```python
from build123d import *

# Parameters (mm, degrees)
SKETCH1_W           = 247.82
SKETCH1_H           = 120.12
SKETCH1_R           = 1.6
SKETCH1_H_2         = 10.57
SKETCH1_H_3         = 1.8
BOSS_EXTRUDE1_DEPTH = 4
SKETCH1_5_W         = 247.82
SKETCH1_5_H         = 1.8
BOSS_EXTRUDE2_DEPTH = 0.8
SKETCH1_6_W         = 247.82
SKETCH1_6_H         = 10.57
BOSS_EXTRUDE3_DEPTH = 1.4
SKETCH2_R           = 2.75
CUT_EXTRUDE1_DEPTH  = 2.9
CUT_EXTRUDE2_REACH  = 287.106
FILLET1_R           = 3


with BuildPart() as part:
    # Sketch1 → Boss-Extrude1 (new body)
    # profile 1 of 5: a face of its own
    with BuildSketch(Plane(origin=(0, 0, 0), x_dir=(1, 0, 0), z_dir=(0, 1, 0))):
        with Locations((126.21, -61.86)):
            Rectangle(SKETCH1_W, SKETCH1_H)
        with Locations(Location((8, -111.92, 0), (0, 0, 270))):
            Circle(SKETCH1_R, mode=Mode.SUBTRACT)
        with Locations(Location((244.42, -111.92, 0), (0, 0, 270))):
            Circle(SKETCH1_R, mode=Mode.SUBTRACT)
        with Locations(Location((8, -61.92, 0), (0, 0, 270))):
            Circle(SKETCH1_R, mode=Mode.SUBTRACT)
        with Locations(Location((8, -8, 0), (0, 0, 270))):
            Circle(SKETCH1_R, mode=Mode.SUBTRACT)
        with Locations(Location((63.11, -8, 0), (0, 0, 270))):
            Circle(SKETCH1_R, mode=Mode.SUBTRACT)
        with Locations(Location((244.42, -61.92, 0), (0, 0, 270))):
            Circle(SKETCH1_R, mode=Mode.SUBTRACT)
        with Locations(Location((126.21, -8, 0), (0, 0, 270))):
            Circle(SKETCH1_R, mode=Mode.SUBTRACT)
        with Locations(Location((189.31, -8, 0), (0, 0, 270))):
            Circle(SKETCH1_R, mode=Mode.SUBTRACT)
        with Locations(Location((244.42, -8, 0), (0, 0, 270))):
            Circle(SKETCH1_R, mode=Mode.SUBTRACT)
    # profile 2 of 5: a face of its own
    with BuildSketch(Plane(origin=(0, 0, 0), x_dir=(1, 0, 0), z_dir=(0, 1, 0))):
        Polygon((252.42, 0), (250.12, 0), (250.12, -1.8), (250.12, -121.92), (250.12, -132.49), (252.42, -132.49), align=None)
    # profile 3 of 5: a face of its own
    with BuildSketch(Plane(origin=(0, 0, 0), x_dir=(1, 0, 0), z_dir=(0, 1, 0))):
        with Locations((126.21, -127.205)):
            Rectangle(SKETCH1_W, SKETCH1_H_2)
    # profile 4 of 5: a face of its own
    with BuildSketch(Plane(origin=(0, 0, 0), x_dir=(1, 0, 0), z_dir=(0, 1, 0))):
        Polygon((2.3, 0), (0, 0), (0, -132.49), (2.3, -132.49), (2.3, -121.92), (2.3, -1.8), align=None)
    # profile 5 of 5: a face of its own
    with BuildSketch(Plane(origin=(0, 0, 0), x_dir=(1, 0, 0), z_dir=(0, 1, 0))):
        with Locations((126.21, -0.9)):
            Rectangle(SKETCH1_W, SKETCH1_H_3)
    extrude(amount=BOSS_EXTRUDE1_DEPTH)

    # Sketch1<5> → Boss-Extrude2 (add)
    with BuildSketch(Plane(origin=(0, 0, 0), x_dir=(1, 0, 0), z_dir=(0, 1, 0))):
        Polygon((2.3, 0), (0, 0), (0, -132.49), (2.3, -132.49), (2.3, -121.92), (2.3, -1.8), align=None)
        with Locations((126.21, -0.9)):
            Rectangle(SKETCH1_5_W, SKETCH1_5_H)
        Polygon((252.42, 0), (250.12, 0), (250.12, -1.8), (250.12, -121.92), (250.12, -132.49), (252.42, -132.49), align=None)
    extrude(amount=-BOSS_EXTRUDE2_DEPTH)

    # Sketch1<6> → Boss-Extrude3 (add)
    with BuildSketch(Plane(origin=(0, 0, 0), x_dir=(1, 0, 0), z_dir=(0, 1, 0))):
        with Locations((126.21, -127.205)):
            Rectangle(SKETCH1_6_W, SKETCH1_6_H)
    extrude(amount=BOSS_EXTRUDE3_DEPTH)

    # Sketch2 → Cut-Extrude1 (cut)
    with BuildSketch(Plane(origin=(0, 4, 0), x_dir=(1, 0, 0), z_dir=(0, 1, 0))):
        with Locations(Location((8, -8, 0), (0, 0, 270))):
            Circle(SKETCH2_R)
        with Locations(Location((63.11, -8, 0), (0, 0, 270))):
            Circle(SKETCH2_R)
        with Locations(Location((126.21, -8, 0), (0, 0, 270))):
            Circle(SKETCH2_R)
        with Locations(Location((189.31, -8, 0), (0, 0, 270))):
            Circle(SKETCH2_R)
        with Locations(Location((244.42, -8, 0), (0, 0, 270))):
            Circle(SKETCH2_R)
        with Locations(Location((244.42, -61.92, 0), (0, 0, 270))):
            Circle(SKETCH2_R)
        with Locations(Location((244.42, -111.92, 0), (0, 0, 270))):
            Circle(SKETCH2_R)
        with Locations(Location((8, -111.92, 0), (0, 0, 270))):
            Circle(SKETCH2_R)
        with Locations(Location((8, -61.92, 0), (0, 0, 270))):
            Circle(SKETCH2_R)
    extrude(amount=-CUT_EXTRUDE1_DEPTH, mode=Mode.SUBTRACT)

    # Sketch3 → Cut-Extrude2 (cut, up to next)
    with BuildSketch(Plane.ZY, mode=Mode.PRIVATE) as cut_extrude2_sk1:
        Polygon((117.49, 4), (132.49, 1), (132.49, 4), align=None)
    cut_extrude2_tool1 = extrude(cut_extrude2_sk1.sketch, amount=-CUT_EXTRUDE2_REACH, mode=Mode.PRIVATE) & part.part
    add(cut_extrude2_tool1.solids().sort_by_distance((0, 3, 127.49))[0], mode=Mode.SUBTRACT)

    # Fillet1
    fillet1_edges = [part.edges().sort_by_distance(p)[0] for p in [
        (0, 4, 58.745),
        (126.21, 4, 0),
        (126.21, 4, 117.49),
        (252.42, 4, 58.745),
    ]]
    fillet(fillet1_edges, radius=FILLET1_R - 0.0001)  # a hair under: the kernel refuses the full size


solid = part.part
```
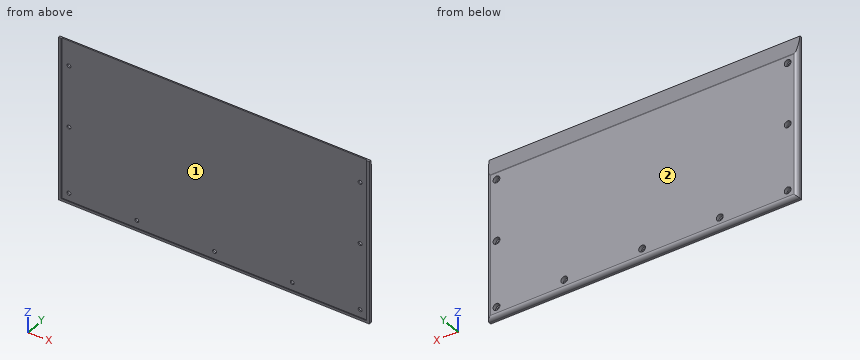
CAD build for the part. Positions are in the model's coordinates, mm. Face numbers are marked on the shaded views. A direction names the side the tool comes from. Coordinates: 2 decimals unless noted, no trailing zeros. Order: outer loops, then holes, each group sorted by start corner. A loop starts at its lowest first (then second) coordinate and runs counter-clockwise, first axis right, second up. Notation, with made-up numbers: (63.5, 52.5) - (72.5, 52.5) arc R24 ccw to (72.5, 68.5) - close; hole circle Ø1 at (77.5, -24). An arc over 180 degrees is marked (long way). Use a Markdown table: item, result. Add a question column.
(1) Saw through at A-A (z = 44). Give the cut face in (x, y).
(2) Saw through at C-C (y = 3.15). Count the separate pieces of the cut face and the enclosed holes in it, then the cut area to 3 significant figures.
(3) Saw through at B-B (x = 29.5). Give the cut face in (y, z).
(4) Flat gauge pins, fed straight in: pin 1 (3.5 mm diameter, centred on x = 126.21, z = 8, fed in from -Y); pin 2 (1 mm diameter, centred on y = 3, z = 86.5, fed in from -X); pin 3 (1.6 mm diameter, centred on x = 7, z = 63, fed in from +Y). Where does each tip first touch, or does it go through?
(5) Which spindle directions (+Z, -Z, +X, -X, +Y, -Y) get a long thin tool onto all of the face, cutting with end or side? Do the marked faces 1 and 2. Say none if no direction does.
(6) Drill centre lines: line 1 along X through (y, z) = (0.55, 8); line 2 along Z through (x, y) = (8, 0.4); line 3 along X through (y, z) = (0.7, 111.92). Where is each one in solid material? Low to high. Write a range as [from, to].
Solved:
| question | item | result |
|---|---|---|
| 1 | outline | (0, -0.8) - (2.3, -0.8) - (2.3, 0) - (250.12, 0) - (250.12, -0.8) - (252.42, -0.8) - (252.42, 1) arc R3 ccw to (249.42, 4) - (3, 4) arc R3 ccw to (0, 1) - close |
| 2 | separate pieces | 1 |
| 2 | enclosed holes | 9 |
| 2 | area | 30,100 mm² |
| 3 | outline | (-0.8, 0) - (1, 0) arc R3 ccw to (4, 3) - (4, 117.19) arc R3 ccw to (3.94, 117.78) - (1, 132.49) - (0, 132.49) - (0, 1.8) - (-0.8, 1.8) - close |
| 4 | pin 1 | stops at y = 0 |
| 4 | pin 2 | stops at x = 0.4 |
| 4 | pin 3 | stops at y = 1.1 |
| 5 | face 1 | +Z, -Y |
| 5 | face 2 | +Z, -Z, +X, -X, +Y |
| 6 | line 1 | x = [0, 6.4], [9.6, 61.51], [64.71, 124.61], [127.81, 187.71], [190.91, 242.82], [246.02, 252.42] |
| 6 | line 2 | z = [0, 6.4], [9.6, 60.32], [63.52, 110.32], [113.52, 132.49] |
| 6 | line 3 | x = [0, 6.4], [9.6, 242.82], [246.02, 252.42] |
